Answer from the drawing. Dimensions are ordinates in mm from the lowest x, y and z of the part. A direction names the side the tool comes from. Give positions to 0.01 mm unless a question says otherwise; leave off trailing zeros. Loops run counter-clockwise (first coordinate to the right, second up) from the corner with the lowest first, then second, coordinate; pieces in that order, holes last. Notation, with made-up numbers: (-24, 24) - (10, 24) arc R11 ccw to (10, 38) - close; hole circle Ø10 at (14.25, 89). An arc over 180 degrees is marked (long way). One line per item, written item: value.
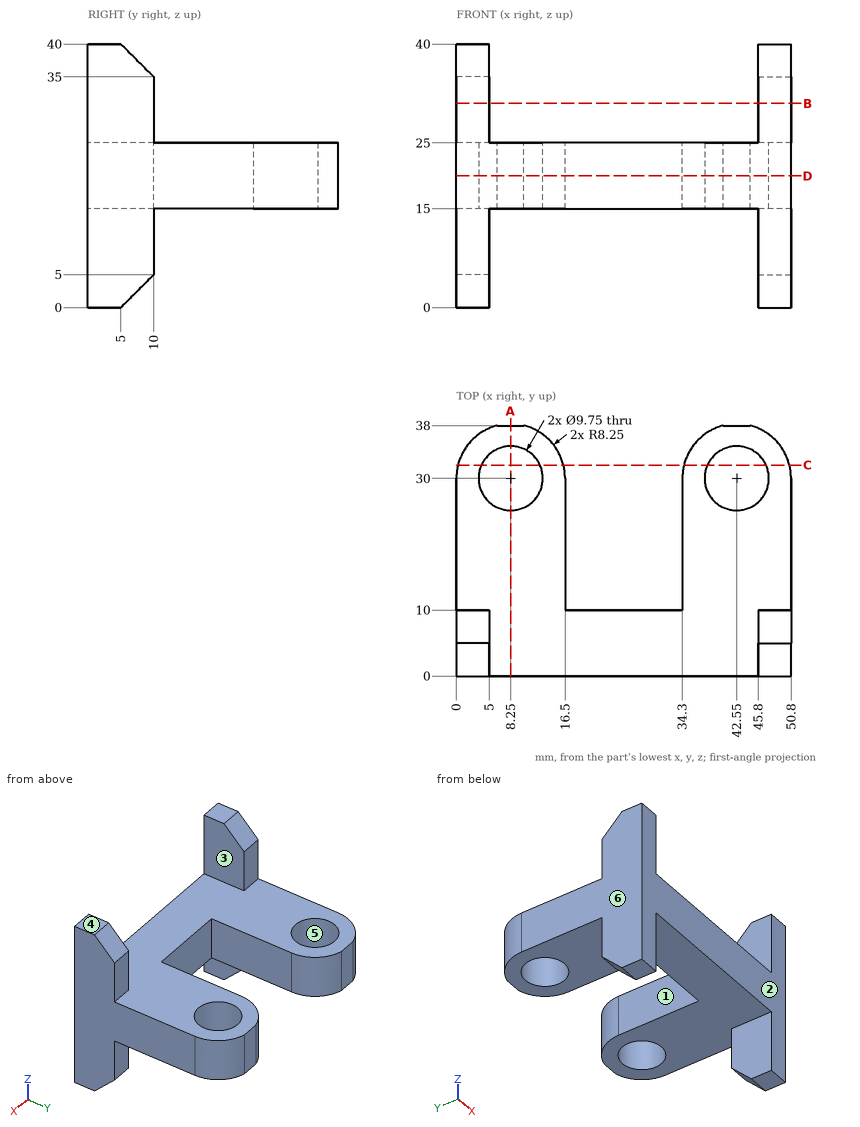
1. Section A-A (x = 8.25) is taken. Write down the section's boundary in (y, z) (3 decimals), and give its area (4 significant figures).
Output:
outline: (0, 15) - (25.125, 15) - (25.125, 25) - (0, 25) - close; (34.875, 15) - (38, 15) - (38, 25) - (34.875, 25) - close
area: 282.5 mm²
2. Section C-C (y = 32) is taken. Write down the section's boundary in (x, z), and give its area (3 significant figures).
Output:
outline: (0.25, 15) - (3.8, 15) - (3.8, 25) - (0.25, 25) - close; (12.7, 15) - (16.25, 15) - (16.25, 25) - (12.7, 25) - close; (34.55, 15) - (38.1, 15) - (38.1, 25) - (34.55, 25) - close; (47, 15) - (50.55, 15) - (50.55, 25) - (47, 25) - close
area: 142 mm²
3. For the marked faces 1, 2 and 3, determine the directions among +Z, -Z, +X, -X, +Y, -Y from which every point of the face is accessible in a straight line to the end or side of a thin tool.
Output:
face 1: +Z, -Z, +Y
face 2: +Z, -Z, +X, -X, -Y
face 3: +Z, +Y, -Y
4. Section B-B (z = 31) is taken. Write down the section's boundary in (x, y), and give its area (3 significant figures).
Output:
outline: (0, 0) - (5, 0) - (5, 10) - (0, 10) - close; (45.8, 0) - (50.8, 0) - (50.8, 10) - (45.8, 10) - close
area: 100 mm²
5. Section D-D (z = 20) is taken. Write down the section's boundary in (x, y) (3 decimals).
Output:
outline: (0, 0) - (50.8, 0) - (50.8, 30) arc R8.25 ccw to (44.566, 38) - (40.534, 38) arc R8.25 ccw to (34.3, 30) - (34.3, 10) - (16.5, 10) - (16.5, 30) arc R8.25 ccw to (10.266, 38) - (6.234, 38) arc R8.25 ccw to (0, 30) - close; hole circle Ø9.75 at (8.25, 30); hole circle Ø9.75 at (42.55, 30)
6. Find the intervals of material crossed by line 1 along Y through (x, z) = (42.55, 17.75) (3 decimals); line 2 along X through (y, z) = (29, 24.5); line 3 along Z through (x, y) = (42.5, 36.5), in increasing order.
Output:
line 1: y = 0 to 25.125, 34.875 to 38
line 2: x = 0 to 3.48, 13.02 to 16.5, 34.3 to 37.78, 47.32 to 50.8
line 3: z = 15 to 25
7. The mould has two halves that part along X. Classify the marked faces 4, 5 and 6: released by +X, released by -X, zero draft, split by the parting line, or undercut.
Output:
face 4: zero draft
face 5: undercut
face 6: released by -X
8. Flat-ended cylindrical pins translate along their axes: pin 1 Ø1.5 at (x, z) = (1.5, 29) entering from +Y; pin 2 Ø10 at (x, z) = (16.5, 9) entering from -Y; pin 3 Ø5 at (y, z) = (5, 4) entering from -X; pin 4 Ø19 at (x, y) = (26, 13) entering from +Z. Find the tip coordinate at first contact, or state that the pin passes through.
Output:
pin 1: stops at y = 10
pin 2: passes through
pin 3: stops at x = 0
pin 4: stops at z = 25
